Geometry: final body of the model. Coordinates: model frame, mm. Coordinates: 2 decimals unless noted, no trailing zeros. Loops run counter-clockwise (first coordinate to the right, second up) from the corner with the lowest first, then second, coordinate; pieces in that order, holes last. Notation, with made-up numbers: (4.5, -15) - (30.5, -15) arc R13 cw to (30.5, 7) - close; hole circle Ø2 at (-23.5, 65). An arc over 180 degrees is marked (long way). Return JSON: item names as keys, results as strings.
from build123d import *

# Parameters (mm, degrees)
CROQUIS2_R              = 0.75
CROQUIS2_W              = 50
CROQUIS2_H              = 50
SALIENTE_EXTRUIR1_DEPTH = 5
CROQUIS3_W              = 6.25
CROQUIS3_H              = 80
CORTAR_EXTRUIR1_DEPTH   = 5


with BuildPart() as part:
    # Croquis2 → Saliente-Extruir1 (new body)
    with BuildSketch(Plane(origin=(0, 0, 0), x_dir=(1, 0, 0), z_dir=(0, 1, 0))):
        Polygon((-62.5, 0), (-62.5, 55), (-55, 62.5), (55, 62.5), (62.5, 55), (62.5, -55), (55, -62.5), (-55, -62.5), (-62.5, -55), align=None)
        with Locations(Location((30, 30, 0), (0, 0, 270))):
            Circle(CROQUIS2_R, mode=Mode.SUBTRACT)
        with Locations(Location((30, 0, 0), (0, 0, 270))):
            Circle(CROQUIS2_R, mode=Mode.SUBTRACT)
        with Locations(Location((30, -30, 0), (0, 0, 270))):
            Circle(CROQUIS2_R, mode=Mode.SUBTRACT)
        with Locations(Location((-30, -30, 0), (0, 0, 270))):
            Circle(CROQUIS2_R, mode=Mode.SUBTRACT)
        with Locations(Location((0, -30, 0), (0, 0, 270))):
            Circle(CROQUIS2_R, mode=Mode.SUBTRACT)
        with Locations(Location((-30, 0, 0), (0, 0, 270))):
            Circle(CROQUIS2_R, mode=Mode.SUBTRACT)
        with Locations(Location((-30, 30, 0), (0, 0, 270))):
            Circle(CROQUIS2_R, mode=Mode.SUBTRACT)
        with Locations(Location((0, 30, 0), (0, 0, 270))):
            Circle(CROQUIS2_R, mode=Mode.SUBTRACT)
        Rectangle(CROQUIS2_W, CROQUIS2_H, mode=Mode.SUBTRACT)
    extrude(amount=SALIENTE_EXTRUIR1_DEPTH)

    # Croquis3 → Cortar-Extruir1 (cut)
    with BuildSketch(Plane(origin=(0, 5, 0), x_dir=(1, 0, 0), z_dir=(0, 1, 0))):
        with Locations((59.375, 0)):
            Rectangle(CROQUIS3_W, CROQUIS3_H)
        with Locations((-59.375, 0)):
            Rectangle(CROQUIS3_W, CROQUIS3_H)
    extrude(amount=-CORTAR_EXTRUIR1_DEPTH, mode=Mode.SUBTRACT)


solid = part.part
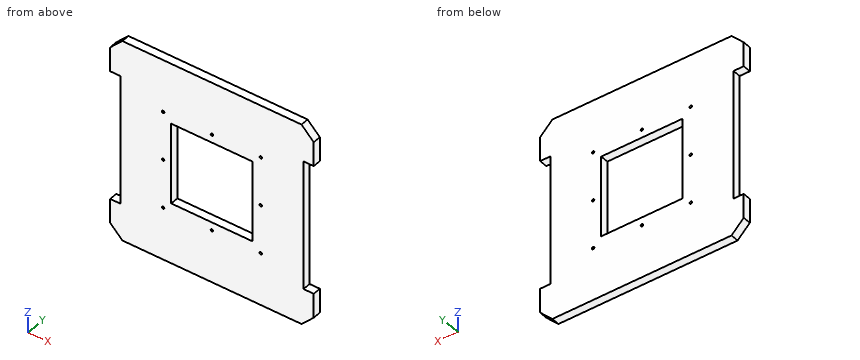
Item 1: Section query C-C, the plane x = -8.5. Return loops of the section in (y, z).
Worked out:
{"outline": "(0, -62.5) - (5, -62.5) - (5, -25) - (0, -25) - close; (0, 25) - (5, 25) - (5, 62.5) - (0, 62.5) - close"}
Item 2: Section query A-A, the plane z = 17.5. Return loops of the section in (x, y), and give its area (4 significant figures).
Worked out:
{"outline": "(-56.25, 0) - (-25, 0) - (-25, 5) - (-56.25, 5) - close; (25, 0) - (56.25, 0) - (56.25, 5) - (25, 5) - close", "area": "312.5 mm^2"}
Item 3: Ray query, probe 1 along X at (y, z) = (1.8, -22); probe 2 along Z at (x, y) = (-19.5, 1.05); probe 3 along X at (y, z) = (3.1, -30). Return the intervals inside material, ascending. Write a range as from..to.
Worked out:
{"probe 1": "-56.25..-25, 25..56.25", "probe 2": "-62.5..-25, 25..62.5", "probe 3": "-56.25..-30.75, -29.25..-0.75, 0.75..29.25, 30.75..56.25"}
Item 4: Section query B-B, the plane y = 0.95. Count the separate pieces of the cut face and the enclosed holes in it, and give its area (3 significant figures).
Worked out:
{"separate pieces": "1", "enclosed holes": "9", "area": "12,000 mm^2"}
Item 5: Section query D-D, the plane z = 37.5. Return loops of the section in (x, y), and give its area (4 significant figures).
Worked out:
{"outline": "(-56.25, 0) - (56.25, 0) - (56.25, 5) - (-56.25, 5) - close", "area": "562.5 mm^2"}
Item 6: First-contact query: pin 1 Ø3 at (y, z) = (3, 18) entering from -X; pin 2 Ø1.5 at (x, y) = (60.5, 1.5) entering from +Z; pin 3 Ø1.5 at (y, z) = (1.5, 0) entering from +X. Flat tips, straight axial feed; report the tip coordinate or a pass-through.
Worked out:
{"pin 1": "x = -56.25", "pin 2": "z = 57.75", "pin 3": "x = 56.25"}
